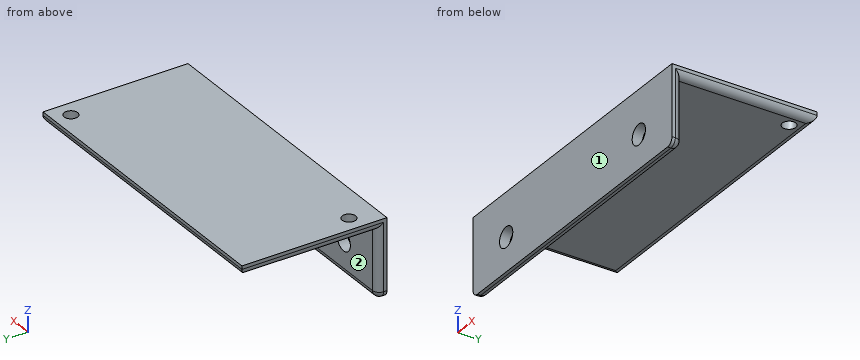
```python
from build123d import *

# Parameters (mm, degrees)
SKETCH1_W           = 45
SKETCH1_H           = 20
SKETCH1_R           = 1
BOSS_EXTRUDE1_DEPTH = 1.5
SKETCH2_W           = 45
SKETCH2_H           = 11.5
SKETCH2_R           = 1.5
BOSS_EXTRUDE2_DEPTH = 1.5
FILLET1_R           = 1


with BuildPart() as part:
    # Sketch1 → Boss-Extrude1 (new body)
    with BuildSketch(Plane.XY):
        Rectangle(SKETCH1_W, SKETCH1_H)
        with Locations((20, 7.5)):
            Circle(SKETCH1_R, mode=Mode.SUBTRACT)
        with Locations((-20, -7.5)):
            Circle(SKETCH1_R, mode=Mode.SUBTRACT)
    extrude(amount=BOSS_EXTRUDE1_DEPTH)

    # Sketch2 → Boss-Extrude2 (add)
    with BuildSketch(Plane.XZ.offset(10)):
        with Locations((0, -4.25)):
            Rectangle(SKETCH2_W, SKETCH2_H)
        with Locations((-15, -5)):
            Circle(SKETCH2_R, mode=Mode.SUBTRACT)
        with Locations((15, -5)):
            Circle(SKETCH2_R, mode=Mode.SUBTRACT)
    extrude(amount=BOSS_EXTRUDE2_DEPTH)

    # Fillet1
    fillet1_edges = [part.edges().sort_by_distance(p)[0] for p in [
        (22.5, -10, -5),
        (22.5, -10.75, -10),
        (-22.5, -10, -5),
        (0, -10, -10),
        (-22.5, -10.75, -10),
        (0, 10, 0),
        (22.5, 0, 0),
        (-22.5, 0, 0),
    ]]
    fillet(fillet1_edges, radius=FILLET1_R)


solid = part.part
```
Here's how the part is built. I have some questions about the finished solid (model axes, mm). Face numbers are marked on the shaded views. A direction names the side the tool comes from. Coordinates: 2 decimals unless noted, no trailing zeros. Write each loop counter-clockwise with the first axis right and the second up, starting at its lowest first coordinate (ties: lowest second). Pieces come first, ordered by that corner, then holes. Notation, with made-up numbers: (-38.75, 52.5) - (5.25, 52.5) arc R7 ccw to (5.25, 65.5) - close; hole circle Ø3 at (-5, 2). An arc over 180 degrees is marked (long way). One line per item, written item: value.
1) On a 3-axis mill with a long thin cutter (end or side, diameter ignored), from which of +Z, -Z, +X, -X, +Y, -Y can I reach the whole of each face in a straight line? I mean the marked faces 1 and 2. Say none if no direction works.
Model answer:
face 1: +Z, -Z, +X, -X, -Y
face 2: -Z, +X, -X, +Y
2) Suppose I cut it at B-B on x = 15. Write out the boundary of the cut face in (y, z), and give its area (3 significant figures).
Model answer:
outline: (-11.5, -10) - (-11, -10) arc R1 ccw to (-10, -9) - (-10, -6.5) - (-11.5, -6.5) - close; (-11.5, -3.5) - (-10, -3.5) - (-10, 0) - (9, 0) arc R1 ccw to (10, 1) - (10, 1.5) - (-11.5, 1.5) - close
area: 42.3 mm²
3) Suppose I cut it at A-A on y = 7.5. Write out the boundary of the cut face in (x, z), and give its area (3 significant figures).
Model answer:
outline: (-22.5, 1) arc R1 ccw to (-21.5, 0) - (19, 0) - (19, 1.5) - (-22.5, 1.5) - close; (21, 0) - (21.5, 0) arc R1 ccw to (22.5, 1) - (22.5, 1.5) - (21, 1.5) - close
area: 64.1 mm²
4) Suppose I cut it at C-C on z = -5. Write out the boundary of the cut face in (x, y).
Model answer:
outline: (-22.5, -11.5) - (-16.5, -11.5) - (-16.5, -10) - (-21.5, -10) arc R1 ccw to (-22.5, -11) - close; (-13.5, -11.5) - (13.5, -11.5) - (13.5, -10) - (-13.5, -10) - close; (16.5, -11.5) - (22.5, -11.5) - (22.5, -11) arc R1 ccw to (21.5, -10) - (16.5, -10) - close
5) I'm going to push flat-ended pins straight in: P1, Ø5, axis at x = -3, y = 6.5, coming from the -Z side; P2, Ø5, axis at y = -2, z = -2, coming from the +X side; P3, Ø2.5, axis at x = -15, z = -5, coming from the -Y side; P4, Ø3, axis at x = 20, y = 7.5, coming from the +Z side. Where does each tip first touch, or does it pass through?
Model answer:
P1: stops at z = 0
P2: stops at x = 22.37
P3: passes through
P4: stops at z = 1.5
6) Suppose I cut it at D-D on y = 1.75. Write out the boundary of the cut face in (x, z).
Model answer:
outline: (-22.5, 1) arc R1 ccw to (-21.5, 0) - (21.5, 0) arc R1 ccw to (22.5, 1) - (22.5, 1.5) - (-22.5, 1.5) - close
7) I need wall thicknesses on line 1 along Y through (x, z) = (-20, 1.05); line 2 along Z through (x, y) = (-19, -1.5); line 3 along Y through (x, z) = (-14, -7). Which ranges of each line are inside material? Lowest first, please.
Model answer:
line 1: y = -11.5 to -8.5, -6.5 to 10
line 2: z = 0 to 1.5
line 3: y = -11.5 to -10
